Geometry: see drawing. Coordinates: mm, zero at the bounding-box minimum. A direction names the side the tool comes from. Give positions to 0.01 mm unless a question says otherwise; leave off trailing zeros. Write each loop counter-clockwise with the first axis right and the second up, starting at its lowest first coordinate (ties: lowest second). Pieces come first, ordered by that corner, then holes. Notation, with made-up numbers: M 76.25,-32 L 102.25,-32 A9 cw 102.25,-17 Z; hole C 60.5,16 d11. An arc over 180 degrees is marked long. Answer as a JSON object with one key per item and string values. Group by question number.
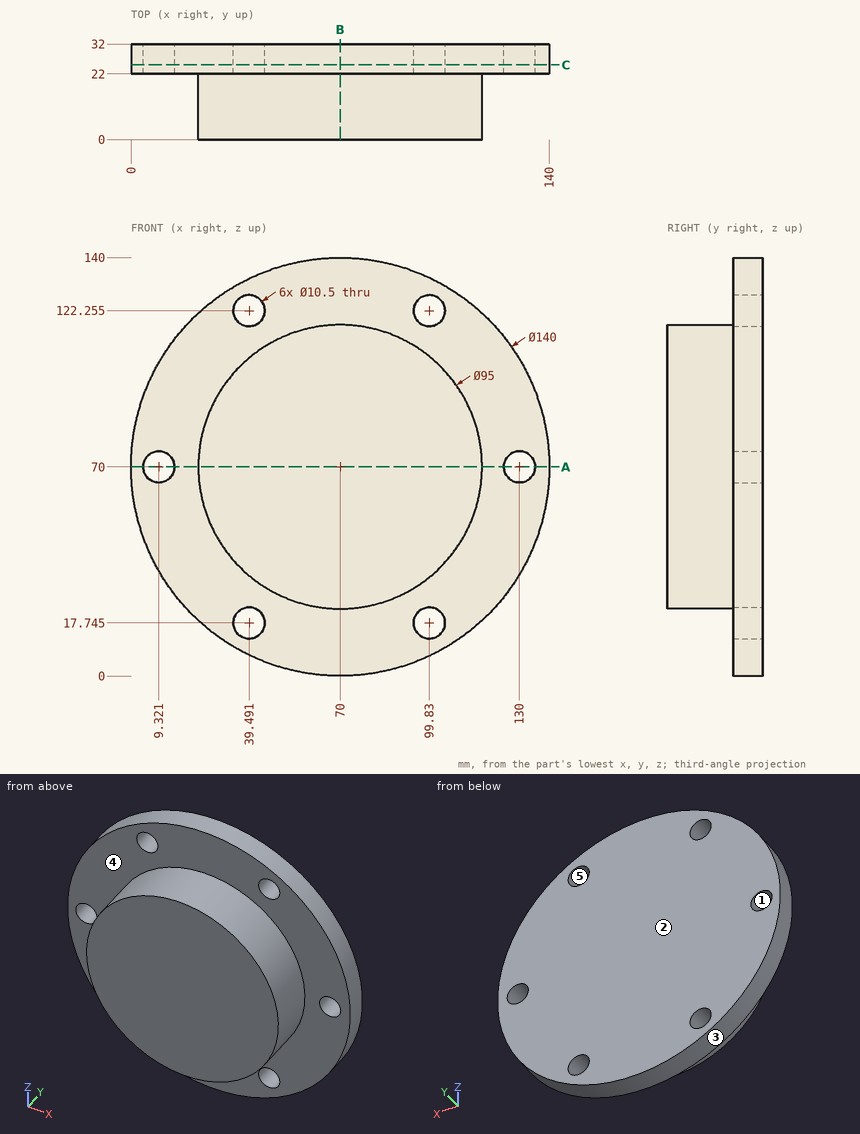
(1) Contact query for flat-ended pins moving along their axis: pin 1 Ø4 at (y, z) = (7, 54) entering from +X; pin 2 Ø10 at (y, z) = (26, 104) entering from -X; pin 3 Ø3 at (y, z) = (22, 87.5) entering from -X. Output: stop coordinate, or through.
(2) Section C-C, the plane y = 25. State how many separate pieces and enclosed holes the cut face has, plus the area to 3 significant figures.
(3) Access query for the marked faces 4 and 5. Directions: +Z, -Z, +X, -X, +Y, -Y. A direction counts if a zero-diameter tool reaches every point of the face in a straight line with its end or side. Return the directions, or none.
(4) Pull-direction query (X, two-part tool) for the marked faces 1, 2 and 3; classes: pulls with the +X half, pulls with the -X half, needs draft (parallel to the pull), parting line crosses it, or undercut.
(5) Section A-A, the plane z = 70. Return loops of the section in (x, y).
(6) Ray query, L1, parallel to X at y = 29, z = 70; L2, parallel to Z at x = 38.5, y = 30.5; L3, parallel to Y at x = 113.5, z = 109. Return the intervals inside material, ascending. Write a range as [from, to].
(7) Section B-B, the plane x = 70. Return loops of the section in (y, z), plus the area to 3 significant figures.
Reported:
{
 "1": {"pin 1": "stops at x = 115.39", "pin 2": "stops at x = 6.29", "pin 3": "stops at x = 1.85"},
 "2": {"separate pieces": "1", "enclosed holes": "6", "area": "14,900 mm2"},
 "3": {"face 4": "-Y", "face 5": "+Y, -Y"},
 "4": {"face 1": "undercut", "face 2": "needs draft", "face 3": "parting line crosses it"},
 "5": {"outline": "M 0,22 L 4.07,22 L 4.07,32 L 0,32 Z; M 14.57,22 L 22.5,22 L 22.5,0 L 117.5,0 L 117.5,22 L 124.75,22 L 124.75,32 L 14.57,32 Z; M 135.25,22 L 140,22 L 140,32 L 135.25,32 Z"},
 "6": {"L1": "x = [0, 4.07], [14.57, 124.75], [135.25, 140]", "L2": "z = [7.49, 12.59], [22.9, 117.1], [127.41, 132.51]", "L3": "y = [22, 32]"},
 "7": {"outline": "M 0,22.5 L 22,22.5 L 22,0 L 32,0 L 32,140 L 22,140 L 22,117.5 L 0,117.5 Z", "area": "3,490 mm2"}
}
